Solid Edge part; units mm, degrees
sketch "Sketch1" plane through (0, 0, 0) normal (0, -1, 0) x (1, 0, 0)
  circle A0 centre (0, 0) radius 6.5
  circle A1 centre (0, 0) radius 8.5
extrude "Protrusion1" add sketch "Sketch1" along normal mid plane 30
fillet "Verrundung_1" radius 1.75 2 edges at (-8.5, 15, 0) (-8.5, -15, 0)
hole "Bohrung_2" at (0, 9, 8.5) direction (0, 0, -1) diameter 3.6 end up to next countersink diameter 6.5 countersink angle 90
properties material "Aluminiumlegierung:3.0205, Al 99.0, EN-AW 1200"
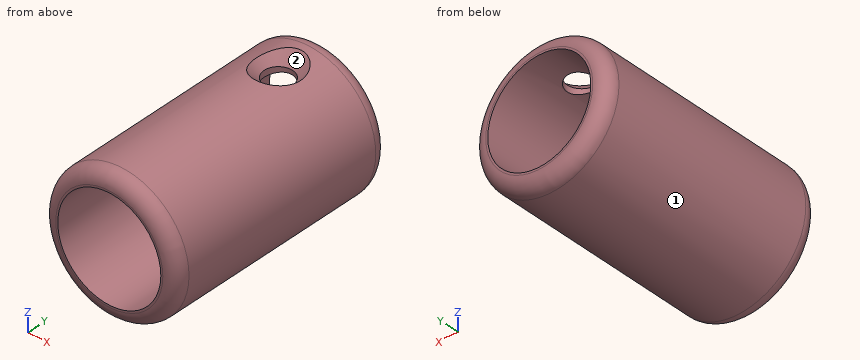
For this review, take the finished solid that the model builds, in its own axes (mm). Face numbers are marked on the shaded views. Give positions to 0.01 mm unless a question says otherwise; leave off trailing zeros. Loops run counter-clockwise (first coordinate to the right, second up) from the corner with the lowest first, then second, coordinate; pieces in that order, holes last. Notation, with made-up numbers: M -3.75,-30.75 L 11.25,-30.75 A26 ccw 11.25,-3.75 Z; hole C 54.5,-9.75 d7. An arc over 180 degrees is marked long. Answer as a JSON object with one key per item and string values. Group by question number.
Q1. Add section A-A on z = 0. Give the boundary of the cut face in (x, y).
Q2. Insertion check: P1, Ø6, axis at x = 0, y = 9, coming from the +Z side; P2, Ø1, axis at y = -5.5, z = -0.5, coming from the -X side; P3, Ø3, axis at x = 3.5, y = 7.5, coming from the -Z side; P4, Ø1.5, axis at x = -4.5, y = 6, coming from the +Z side. Each pin has a flat end and moves straight along its axis. Give the tip position at first contact, or say it passes through.
Q3. Add section D-D on y = 9. Give the boundary of the cut face in (x, z).
Q4. Add section B-B on x = 0. Give the boundary of the cut face in (y, z), and give its area (3 significant figures).
Q5. Add section C-C on y = -6. Give the boundary of the cut face in (x, z), and give its area (3 significant figures).
Q6. Mouldability with a two-part tool opening along X and no side actions: class the marked faces 1 and 2 as +X half, -X half, draft (parallel to the pull), parting line (faces both ways), or undercut.
Q7. For probe 1 along Y at (x, z) = (-1.25, 7.25); probe 2 along X at (y, z) = (5, 6); probe 3 along Z at (x, y) = (-2.5, -6.5), list the stretches that pass through material, from the lowest coordinate up. Write a range as [from, to].
Checked values:
{
 "1": {"outline": "M -8.5,-13.25 A1.75 ccw -6.75,-15 L -6.5,-15 L -6.5,15 L -6.75,15 A1.75 ccw -8.5,13.25 Z; M 6.5,-15 L 6.75,-15 A1.75 ccw 8.5,-13.25 L 8.5,13.25 A1.75 ccw 6.75,15 L 6.5,15 Z"},
 "2": {"P1": "z = 8.25", "P2": "x = -8.5", "P3": "z = -8.26", "P4": "z = 7.63"},
 "3": {"outline": "M -2.78,8.03 A8.5 ccw long 2.78,8.03 L 1.8,7.05 L 1.8,6.25 A6.5 cw long -1.8,6.25 L -1.8,7.05 Z"},
 "4": {"outline": "M -15,-6.75 A1.75 ccw -13.25,-8.5 L 13.25,-8.5 A1.75 ccw 15,-6.75 L 15,-6.5 L -15,-6.5 Z; M -15,6.5 L 7.2,6.5 L 7.2,7.05 L 5.75,8.5 L -13.25,8.5 A1.75 ccw -15,6.75 Z; M 10.8,6.5 L 15,6.5 L 15,6.75 A1.75 ccw 13.25,8.5 L 12.25,8.5 L 10.8,7.05 Z", "area": "108 mm²"},
 "5": {"outline": "C 0,0 d17; hole C 0,0 d13", "area": "94.2 mm²"},
 "6": {"face 1": "parting line", "face 2": "undercut"},
 "7": {"probe 1": "[-14.89, 7.44], [10.56, 14.89]", "probe 2": "[-6.02, -2.5], [2.5, 6.02]", "probe 3": "[-8.12, -6], [6, 8.12]"}
}
